Can you work these out from the model? Positions are in its coordinate system, mm. A direction names the side the tool comes from. Round coordinates to 2 decimals unless told otherwise and drop trailing zeros. Order: outer loops, then holes, each group sorted by start corner. A loop starts at its lowest first (then second) coordinate and runs counter-clockwise, first axis right, second up. Notation, with made-up numbers: (-3, -6) -> (56, -6) arc R29 cw to (56, 21) -> close; hole circle Ø9 at (48.25, 61.25). An arc over 180 degrees is marked (long way). One line per item, written item: value.
Autodesk Inventor part; units mm, degrees
ref_plane "YZ Plane" through (0, 0, 0) normal (1, 0, 0) x (0, 1, 0)
ref_plane "XZ Plane" through (0, 0, 0) normal (0, 1, 0) x (-1, 0, 0)
ref_plane "XY Plane" through (0, 0, 0) normal (0, 0, 1) x (1, 0, 0)
sketch "スケッチ1" plane through (0, 0, 0) normal (0, 0, 1) x (1, 0, 0)
  line L0 (1.0771, -3.8522) -> (-54.1543, -19.2955)
  line L1 (-60, -27) -> (-63, -27)
  arc A0 (-63, -27) -> (-66, -27) centre (-64.5, -27) ccw
  line L2 (-66, -27) -> (-66, -30)
  line L3 (-66, -30) -> (-80, -30)
  line L4 (-80, -30) -> (-80, -27)
  arc A1 (-80, -27) -> (-83, -27) centre (-81.5, -27) ccw
  line L5 (-83, -27) -> (-86, -27)
  arc A2 (-80.6768, -18.161) -> (-86, -27) centre (-76, -27) ccw
  line L6 (-80.6768, -18.161) -> (-1.8707, 23.5356)
  line L7 (4, 20) -> (4, 0)
  line L8 (-76, -25.5) -> (-70, -25.5) construction
  line L9 (-76, -27) -> (-70, -27)
  line L10 (-70, -24) -> (-76, -24)
  arc A3 (-76, -24) -> (-76, -27) centre (-76, -25.5) ccw
  arc A4 (-70, -27) -> (-70, -24) centre (-70, -25.5) ccw
  circle A5 centre (0, 0) radius 1.6
  circle A6 centre (0, 20) radius 1.6
  arc A7 (1.0771, -3.8522) -> (4, 0) centre (0, 0) ccw
  arc A8 (4, 20) -> (-1.8707, 23.5356) centre (0, 20) ccw
  arc A9 (-54.1543, -19.2955) -> (-60, -27) centre (-52, -27) ccw
  point P0 (-73, -25.5)
  point P1 (-73, -30)
  dimension "d0" = 3
  dimension "d1" = 6
  dimension "d2" = 14
  dimension "d3" = 1.5
  dimension "d4" = 3
  dimension "d5" = 1.5
  dimension "d6" = 3
  dimension "d9" = 3.2
  dimension "d10" = 3.2
  dimension "d13" = 4
  dimension "d14" = 20
  dimension "d15" = 30
  dimension "d16" = 10
  dimension "d19" = 8
  dimension "d20" = 60
extrude "押し出し1" add sketch "スケッチ1" along normal blind 3
equation "\"d6\" = d0"
properties part number "BaseSliderSupport"
Q1. I want a section at D-D on x = -22. List the corners of the cut face in (y, z) for me.
Answers below:
outline: (-10.3, 0) -> (12.89, 0) -> (12.89, 3) -> (-10.3, 3) -> close
Q2. We'd pull the mould along Y, two halves only. Please class faces 6 (the face through (-84.6, -21.9, 1.5)), 7 (the face through (-73, -24, 1)), 8 (the face through (-80, -29, 1)): released by +Y, released by -Y, zero draft, split by the parting line, or undercut.
Answers below:
face 6: released by +Y
face 7: undercut
face 8: zero draft
Q3. I want a section at B-B on x = 0. List the corners of the cut face in (y, z) for me.
Answers below:
outline: (-4.15, 0) -> (-1.6, 0) -> (-1.6, 3) -> (-4.15, 3) -> close; (1.6, 0) -> (18.4, 0) -> (18.4, 3) -> (1.6, 3) -> close; (21.6, 0) -> (24, 0) -> (24, 3) -> (21.6, 3) -> close
Q4. On a 3-axis mill with a long thin cutter (end or side, diameter ignored), from which of +Z, -Z, +X, -X, +Y, -Y can I reach the whole of each face in a straight line? I mean faces 1 (the face through (-66, -28, 1)), 2 (the face through (-35, -5, 0)), 3 (the face through (-64.5, -25.5, 1.5)), 4 (the face through (-68.5, -25.5, 1.5)), 5 (the face through (-84, -27, 1)). Say none if no direction works.
Answers below:
face 1: +Z, -Z, +X, -Y
face 2: -Z, +X, -X, +Y, -Y
face 3: +Z, -Z, -Y
face 4: +Z, -Z
face 5: +Z, -Z, -X, -Y
Q5. I want a section at C-C on y = -7.5. List the corners of the cut face in (x, z) for me.
Answers below:
outline: (-60.53, 0) -> (-11.97, 0) -> (-11.97, 3) -> (-60.53, 3) -> close
Q6. Please list where these lines run through material, in increasing order: line 1 along Y through (x, z) = (0, 2.2); line 2 along X through (y, z) = (19.5, 0.25); line 3 along Y through (x, z) = (-23.5, 0.9).
Answers below:
line 1: -4.15 to -1.6, 1.6 to 18.4, 21.6 to 24
line 2: -9.5 to -1.52, 1.52 to 4
line 3: -10.72 to 12.09
Q7. I want a section at A-A on z = 1.65. List the corners of the cut face in (x, y) for me.
Answers below:
outline: (-86, -27) -> (-83, -27) arc R1.5 cw to (-80, -27) -> (-80, -30) -> (-66, -30) -> (-66, -27) arc R1.5 cw to (-63, -27) -> (-60, -27) arc R8 cw to (-54.15, -19.3) -> (1.08, -3.85) arc R4 ccw to (4, 0) -> (4, 20) arc R4 ccw to (-1.87, 23.54) -> (-80.68, -18.16) arc R10 ccw to start; hole (-76, -27) -> (-70, -27) arc R1.5 ccw to (-70, -24) -> (-76, -24) arc R1.5 ccw to start; hole circle Ø3.2 at (0, 0); hole circle Ø3.2 at (0, 20)
Q8. Will these pins go through, and if not, where does the flat tip stop? pin 1 Ø0.9 at (x, z) = (-84.5, 1.5) entering from -Y; pin 2 Ø1.5 at (y, z) = (-23.5, 2) entering from +X; pin 3 Ø0.9 at (x, z) = (-73, 1.5) entering from +Y.
Answers below:
pin 1: y = -27
pin 2: x = -58.78
pin 3: y = -13.86
